Input: dimensioned drawing with shaded views. Units: mm. Origin: part minimum x, y, z. A direction names the side the tool comes from. Give positions to 0.01 mm unless a question says otherwise; leave off trailing zeros. Write each loop counter-clockwise with the first axis right and the second up, starting at its lowest first coordinate (ties: lowest second). Pieces come first, ordered by that corner, then holes.
Q1. Reachability of the marked faces 1, 2 and 3 from +Z, -Z, +X, -X, +Y, -Y: full face, straight path, thin tool, end or side. Return the list, or none.
Q2. Line query: line 1 (Y direction, x = 105, z = 3); line 2 (X direction, y = 15, z = 4.5); line 3 (X direction, y = 19.75, z = 13.25). Output: solid intervals per line, ascending.
Q3. Section B-B (z = 8.25). Return the cut outline in (x, y), plus the area to 3 significant figures.
Q4. Section D-D (y = 15). Return the cut outline in (x, z), plus the area to 3 significant figures.
Q5. Section C-C (y = 5). Return the cut outline in (x, z), plus the area to 3 significant figures.
Q6. Pin query (flat end, axial travel): pin 1 Ø4 at (x, z) = (45.5, 6.5) entering from -Y; pin 2 Ø1.5 at (x, z) = (47, 3) entering from -Y (3 decimals); pin 3 Ø10 at (x, z) = (52, 10.5) entering from +Y. Return the tip coordinate at first contact, or that it passes through.
Q7. Section A-A (x = 105). Return the cut outline in (y, z).
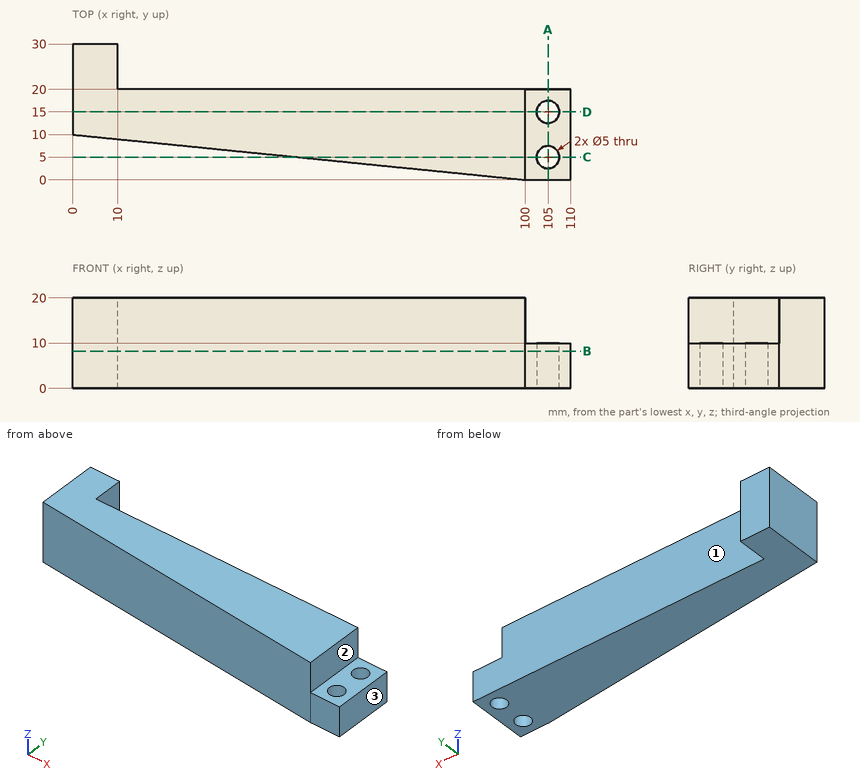
Computed:
1. face 1: +Z, -Z, +X, +Y
1. face 2: +Z, +X, +Y, -Y
1. face 3: +Z, -Z, +X, +Y, -Y
2. line 1: y = 0 to 2.5, 7.5 to 12.5, 17.5 to 20
2. line 2: x = 0 to 102.5, 107.5 to 110
2. line 3: x = 0 to 100
3. outline: (0, 10) - (100, 0) - (110, 0) - (110, 20) - (10, 20) - (10, 30) - (0, 30) - close; hole circle Ø5 at (105, 5); hole circle Ø5 at (105, 15)
3. area: 1,760 mm2
4. outline: (0, 0) - (102.5, 0) - (102.5, 10) - (100, 10) - (100, 20) - (0, 20) - close; (107.5, 0) - (110, 0) - (110, 10) - (107.5, 10) - close
4. area: 2,050 mm2
5. outline: (50, 0) - (102.5, 0) - (102.5, 10) - (100, 10) - (100, 20) - (50, 20) - close; (107.5, 0) - (110, 0) - (110, 10) - (107.5, 10) - close
5. area: 1,050 mm2
6. pin 1: stops at y = 5.25
6. pin 2: stops at y = 5.225
6. pin 3: stops at y = 20
7. outline: (0, 0) - (2.5, 0) - (2.5, 10) - (0, 10) - close; (7.5, 0) - (12.5, 0) - (12.5, 10) - (7.5, 10) - close; (17.5, 0) - (20, 0) - (20, 10) - (17.5, 10) - close
